CAD build for the part. Positions are in the model's coordinates, mm. A direction names the side the tool comes from. Coordinates: 2 decimals unless noted, no trailing zeros. Write each loop counter-clockwise with the first axis right and the second up, starting at its lowest first coordinate (ties: lowest second). Pieces come first, ordered by that corner, then holes.
```python
from build123d import *

# Parameters (mm, degrees)
BOSS_EXTRUDE1_DEPTH      = 225
BOSS_EXTRUDE1_DEPTH_BACK = 225
FILLET1_R                = 13.5
FILLET2_R                = 13.5
FILLET3_R                = 13.5
SKETCH2_R                = 3.75
CUT_EXTRUDE1_DEPTH       = 407.610144979
SKETCH3_R                = 2.217250466
SKETCH3_R_2              = 2.287005769
SKETCH3_R_3              = 2.375
SKETCH3_W                = 13.962530501
SKETCH3_H                = 28.400000001
CUT_EXTRUDE2_DEPTH       = 407.610144979


with BuildPart() as part:
    # Sketch1 → Boss-Extrude1 (new, two sides: drawn at the far end of the back side and taken through both)
    with BuildSketch(Plane.XY.offset(-BOSS_EXTRUDE1_DEPTH_BACK)):
        with BuildLine():
            Line((-329.1, -55), (-329.1, -80))
            Line((-329.1, -80), (-156.365701077, -80))
            ThreePointArc((-156.365701077, -80), (-147.072914305, -76.292554009), (-142.884202358, -67.206535409))
            Line((-142.884202358, -67.206535409), (-139.982869184, -11.845800547))
            ThreePointArc((-139.982869184, -11.845800547), (-136.104432196, -3.432820362), (-127.5, 0))
            Line((-127.5, 0), (127.5, 0))
            ThreePointArc((127.5, 0), (136.104432196, -3.432820362), (139.982869184, -11.845800547))
            Line((139.982869184, -11.845800547), (142.884202358, -67.206535409))
            ThreePointArc((142.884202358, -67.206535409), (147.072914305, -76.292554009), (156.365701077, -80))
            Line((156.365701077, -80), (329.1, -80))
            Line((329.1, -80), (329.1, -55))
            Line((329.1, -55), (179.140850678, -55))
            ThreePointArc((179.140850678, -55), (170.536418482, -51.567179638), (166.657981494, -43.154199453))
            Line((166.657981494, -43.154199453), (163.75664832, 12.206535409))
            ThreePointArc((163.75664832, 12.206535409), (159.567936373, 21.292554009), (150.275149601, 25))
            Line((150.275149601, 25), (-150.275149601, 25))
            ThreePointArc((-150.275149601, 25), (-159.567936373, 21.292554009), (-163.75664832, 12.206535409))
            Line((-163.75664832, 12.206535409), (-166.657981494, -43.154199453))
            ThreePointArc((-166.657981494, -43.154199453), (-170.536418482, -51.567179638), (-179.140850678, -55))
            Line((-179.140850678, -55), (-329.1, -55))
        make_face()
    extrude(amount=BOSS_EXTRUDE1_DEPTH + BOSS_EXTRUDE1_DEPTH_BACK)

    # Fillet1
    fillet1_edges = [part.edges().sort_by_distance(p)[0] for p in [
        (-242.732850539, -80, -225),
        (-147.072914305, -76.292554009, -225),
        (-141.433535771, -39.526167978, -225),
        (-136.104432196, -3.432820362, -225),
        (0, 0, -225),
        (136.104432196, -3.432820362, -225),
        (-329.1, -80, 0),
        (141.433535771, -39.526167978, -225),
        (147.072914305, -76.292554009, -225),
        (242.732850539, -80, -225),
        (-242.732850539, -80, 225),
        (-147.072914305, -76.292554009, 225),
        (-141.433535771, -39.526167978, 225),
        (-136.104432196, -3.432820362, 225),
        (0, 0, 225),
        (136.104432196, -3.432820362, 225),
        (141.433535771, -39.526167978, 225),
        (147.072914305, -76.292554009, 225),
        (242.732850539, -80, 225),
    ]]
    fillet(fillet1_edges, radius=FILLET1_R)

    # Fillet2
    fillet2_edges = [part.edges().sort_by_distance(p)[0] for p in [
        (329.1, -80, 0),
        (329.1, -60.75, 225),
        (329.1, -60.75, -225),
        (329.1, -76.045941546, 221.045941546),
        (329.1, -76.045941546, -221.045941546),
    ]]
    fillet(fillet2_edges, radius=FILLET2_R)

    # Fillet3
    # the kernel refuses this fillet: 13.5 mm, written as the material it takes off along each edge
    with BuildSketch(Plane(origin=(-315.6, -66.5, 211.5), x_dir=(0, 0, 1), z_dir=(-1, 0, 0))) as fillet3_piece_1_section:
        Polygon((0, 0), (FILLET3_R, 0), (FILLET3_R, -FILLET3_R), (0, -FILLET3_R), align=None)
    fillet3_piece_1 = extrude(amount=FILLET3_R, mode=Mode.PRIVATE)
    fillet3_piece_1 = fillet3_piece_1 - Plane(origin=(-315.6, -66.5, 211.5), x_dir=(0, 0.7071067811865475, -0.7071067811865475), z_dir=(-1, 0, 0)) * Sphere(FILLET3_R, mode=Mode.PRIVATE)
    add(fillet3_piece_1, mode=Mode.SUBTRACT)
    with BuildSketch(Plane(origin=(-315.6, -66.5, -211.5), x_dir=(-1, 0, 0), z_dir=(0, 0, -1))) as fillet3_piece_2_section:
        Polygon((0, 0), (FILLET3_R, 0), (FILLET3_R, -FILLET3_R), (0, -FILLET3_R), align=None)
    fillet3_piece_2 = extrude(amount=FILLET3_R, mode=Mode.PRIVATE)
    fillet3_piece_2 = fillet3_piece_2 - Plane(origin=(-315.6, -66.5, -211.5), x_dir=(0.7071067811865475, 0.7071067811865475, 0), z_dir=(0, 0, -1)) * Sphere(FILLET3_R, mode=Mode.PRIVATE)
    add(fillet3_piece_2, mode=Mode.SUBTRACT)
    with BuildSketch(Plane(origin=(-329.1, -21.25, 225), x_dir=(0, 0, -1), z_dir=(0, -1, 0)), Plane(origin=(-329.1, -21.25, -225), x_dir=(1, 0, 0), z_dir=(0, -1, 0))) as fillet3_piece_3:
        with BuildLine():
            CenterArc((FILLET3_R, FILLET3_R), FILLET3_R, 180, 90)
            Line((0, FILLET3_R), (0, 0))
            Line((0, 0), (FILLET3_R, 0))
        make_face()
    extrude(amount=45.25, mode=Mode.SUBTRACT)

    # Sketch2 → Cut-Extrude1 (cut, through all)
    with BuildSketch(Plane(origin=(0, -55, 0), x_dir=(1, 0, 0), z_dir=(0, 1, 0))):
        with Locations(Location((264.653924111, 33.529574354, 0), (0, 0, 180))):
            Circle(SKETCH2_R)
        with Locations(Location((264.653924111, 16.529574354, 0), (0, 0, 180))):
            Circle(SKETCH2_R)
        with Locations(Location((264.805133934, -17, 0), (0, 0, 180))):
            Circle(SKETCH2_R)
        with Locations(Location((264.805133934, -34, 0), (0, 0, 180))):
            Circle(SKETCH2_R)
        with Locations(Location((241.140850678, -195, 0), (0, 0, 180))):
            Circle(SKETCH2_R)
        with Locations(Location((241.140850678, -123.52, 0), (0, 0, 180))):
            Circle(SKETCH2_R)
        with Locations(Location((241.140850678, 123.049574354, 0), (0, 0, 180))):
            Circle(SKETCH2_R)
        with Locations(Location((241.140850678, 194.529574354, 0), (0, 0, 180))):
            Circle(SKETCH2_R)
    extrude(amount=-CUT_EXTRUDE1_DEPTH, mode=Mode.SUBTRACT)

    # Sketch3 → Cut-Extrude2 (cut, through all)
    with BuildSketch(Plane.XZ):
        with Locations((1.08258839, -184.160446131)):
            Circle(SKETCH3_R)
        with Locations((4.060016021, -162.119555044)):
            Circle(SKETCH3_R_2)
        with Locations((-17.624379629, -175.332)):
            Circle(SKETCH3_R_3)
        with Locations((30.315969329, -175.921080945)):
            Rectangle(SKETCH3_W, SKETCH3_H)
    extrude(amount=-CUT_EXTRUDE2_DEPTH, mode=Mode.SUBTRACT)


solid = part.part
```
Item 1: Which spindle directions (+Z, -Z, +X, -X, +Y, -Y) get a long thin tool onto all of the face, cutting with end or side? Do faces 1 (the cylindrical face through (-136.2, -3.525, -2.961)), 2 (the cylindrical face through (-145.26, -38.94, -220.94)), 3 (the flat face through (37.297, 12, -176)). Say none if no direction does.
Item 2: Two-plate mould, pull along X, no slides. Class faces 4 (the flat face through (30, 12, -190.121)), 5 (the cylindrical face through (325.25, -75.94, 2.96)), 6 (the flat face through (-1, 17, 225)): +X half, -X half, draft (parallel to the pull), parting line (faces both ways), or undercut.
Item 3: Wall check: line 1 along Y through (x, z) = (220, -106.5); line 2 along X through (y, z) = (-62, 80.5); line 3 along Y through (x, z) = (-13.5, 66). Give the ranges that are in metal, low to high.
Item 4: Saw through at B-B, the plane x = 277. Write the cut outline in (y, z).
Item 5: Saw through at A-A, the plane z = 77. Write the cut outline in (x, y), and give its area (3 significant figures).
Item 6: Flat gauge pins, fed straight in: pin 1 Ø8.5 at (x, z) = (241.14, -194.53) entering from +Y; pin 2 Ø7.5 at (y, z) = (8.5, -174) entering from +X; pin 3 Ø6 at (y, z) = (-16, 4) entering from -X. Where does each tip first touch, or does it go through?
Working result:
1. face 1: +Z, -Z, -Y
1. face 2: -Z, -Y
1. face 3: +Y, -Y
2. face 4: undercut
2. face 5: +X half
2. face 6: draft
3. line 1: y = -80 to -55
3. line 2: x = -329.1 to -142.61, 142.61 to 329.1
3. line 3: y = 0 to 25
4. outline: (-80, -211.5) arc R13.5 ccw to (-66.5, -225) - (-55, -225) - (-55, 225) - (-66.5, 225) arc R13.5 ccw to (-80, 211.5) - close
5. outline: (-329.1, -66.5) arc R13.5 ccw to (-315.6, -80) - (-156.37, -80) arc R13.5 ccw to (-142.88, -67.21) - (-139.98, -11.85) arc R12.5 cw to (-127.5, 0) - (127.5, 0) arc R12.5 cw to (139.98, -11.85) - (142.88, -67.21) arc R13.5 ccw to (156.37, -80) - (315.6, -80) arc R13.5 ccw to (329.1, -66.5) - (329.1, -55) - (179.14, -55) arc R12.5 cw to (166.66, -43.15) - (163.76, 12.21) arc R13.5 ccw to (150.28, 25) - (-150.28, 25) arc R13.5 ccw to (-163.76, 12.21) - (-166.66, -43.15) arc R12.5 cw to (-179.14, -55) - (-329.1, -55) - close
5. area: 20,200 mm2
6. pin 1: stops at y = -55
6. pin 2: stops at x = 164.15
6. pin 3: stops at x = -165.39
